The model under review builds one solid part; all positions refer to its coordinate system, in mm. A direction names the side the tool comes from. Round coordinates to 2 decimals unless told otherwise and drop trailing zeros. Order: outer loops, then holes, each group sorted by start corner. A loop starts at its lowest first (then second) coordinate and runs counter-clockwise, first axis right, second up.
```python
from build123d import *

# Parameters (mm, degrees)
EXTRUDE_1_DEPTH     = 2
EXTRUDE_2_DEPTH     = 120
SKETCH_3_R          = 5
SKETCH_3_R_2        = 3
CUT_EXTRUDE_1_DEPTH = 2
SKETCH_4_R          = 5
SKETCH_4_R_2        = 3
CUT_EXTRUDE_2_DEPTH = 2
SKETCH_5_R          = 3
CUT_EXTRUDE_3_DEPTH = 2


with BuildPart() as part:
    # 草图1 → 凸台-拉伸1 (new body)
    with BuildSketch(Plane(origin=(0, 0, 0), x_dir=(1, 0, 0), z_dir=(0, 1, 0))):
        with BuildLine():
            Line((-71.645096328, 99.585522078), (-71.645096328, -20.414477922))
            Line((-71.645096328, -20.414477922), (48.354903672, -20.414477922))
            Line((48.354903672, -20.414477922), (48.354903672, -18.414477922))
            Line((48.354903672, -18.414477922), (-1.806261563, 31.746687313))
            ThreePointArc((-1.806261563, 31.746687313), (-19.483931092, 31.746687313), (-19.483931092, 49.424356842))
            Line((-19.483931092, 49.424356842), (-69.645096328, 99.585522078))
            Line((-69.645096328, 99.585522078), (-71.645096328, 99.585522078))
        make_face()
    extrude(amount=EXTRUDE_1_DEPTH)

    # 草图2 → 凸台-拉伸2 (add)
    with BuildSketch(Plane(origin=(0, 2, 0), x_dir=(1, 0, 0), z_dir=(0, 1, 0))):
        Polygon((-69.645096328, 99.585522078), (-69.645096328, -18.414477922), (48.354903672, -18.414477922), (48.354903672, -20.414477922), (-71.645096328, -20.414477922), (-71.645096328, 99.585522078), align=None)
    extrude(amount=EXTRUDE_2_DEPTH)

    # 草图3 → 切除-拉伸1 (cut)
    with BuildSketch(Plane(origin=(0, 0, 18.414477922), x_dir=(-1, 0, 0), z_dir=(0, 0, -1))):
        with Locations((0.645096328, 112)):
            Circle(SKETCH_3_R)
        with Locations((20.645096328, 112)):
            Circle(SKETCH_3_R)
        with Locations((10.645096328, 112)):
            Circle(SKETCH_3_R_2)
    extrude(amount=-CUT_EXTRUDE_1_DEPTH, mode=Mode.SUBTRACT)

    # 草图4 → 切除-拉伸2 (cut)
    with BuildSketch(Plane(origin=(-69.645096328, 0, 0), x_dir=(0, 0, -1), z_dir=(1, 0, 0))):
        with Locations((30.585522078, 112)):
            Circle(SKETCH_4_R)
        with Locations((50.585522078, 112)):
            Circle(SKETCH_4_R)
        with Locations((40.585522078, 111.785381459)):
            Circle(SKETCH_4_R_2)
        with Locations((40.585522078, 104.992052501)):
            Circle(SKETCH_4_R_2)
    extrude(amount=-CUT_EXTRUDE_2_DEPTH, mode=Mode.SUBTRACT)

    # 草图5 → 切除-拉伸3 (cut)
    with BuildSketch(Plane(origin=(0, 0, 18.414477922), x_dir=(-1, 0, 0), z_dir=(0, 0, -1))):
        with Locations((10.645096328, 105)):
            Circle(SKETCH_5_R)
    extrude(amount=-CUT_EXTRUDE_3_DEPTH, mode=Mode.SUBTRACT)


solid = part.part
```
(1) For faces 4 (the flat face through (23.63, 0.99, -6.31)), 5 (the flat face through (-69.645, 61, -41)), list the 3-axis set-ups (+Z, -Z, +X, -X, +Y, -Y) from which the entire face can be reached by the end or side of a thin tool; tool diameter is ignored.
Data:
face 4: -Z, +X, +Y, -Y
face 5: -Z, +X, +Y
(2) Draft analysis for pull direction Y (two halves, no side actions). For faces 1 (the flat face through (-38, 2, -15)), 2 (the cylindrical face through (-19.287, 0.986, -31.554)), 3 (the cylindrical face through (-70.631, 107.967, -40.195)), state which applies: pulls with the +Y half, pulls with the -Y half, needs draft (parallel to the pull), parting line crosses it, or undercut.
Data:
face 1: pulls with the +Y half
face 2: needs draft
face 3: undercut
(3) Consider section A-A (y = 72). Write out the cut boundary in (x, z), and give its area (3 significant figures).
Data:
outline: (-71.65, -99.59) - (-69.65, -99.59) - (-69.65, 18.41) - (48.35, 18.41) - (48.35, 20.41) - (-71.65, 20.41) - close
area: 476 mm2
(4) To check wall thickness, follow probe 1 along Z at (x, y) = (39, 101.5); probe 2 along Y at (x, z) = (-62, -38); probe 3 along X at (y, z) = (102.5, 11). State the ranges of each line that lie inside material, in increasing order.
Data:
probe 1: z = 18.41 to 20.41
probe 2: y = 0 to 2
probe 3: x = -71.65 to -69.65
(5) Insertion check: pin 1 (16 mm diameter, centred on y = 112, z = -50.59, fed in from +X); pin 2 (2 mm diameter, centred on x = -7, y = 100, fed in from -Z); pin 3 (6 mm diameter, centred on x = -0.65, y = 112, fed in from -Z). Each pin has a flat end and moves straight along its axis. Give the tip position at first contact, or say it passes through.
Data:
pin 1: stops at x = -69.65
pin 2: stops at z = 18.41
pin 3: passes through
(6) Consider section B-B (x = -41.5). Write out the cut boundary in (y, z).
Data:
outline: (0, -71.44) - (2, -71.44) - (2, 18.41) - (122, 18.41) - (122, 20.41) - (0, 20.41) - close
